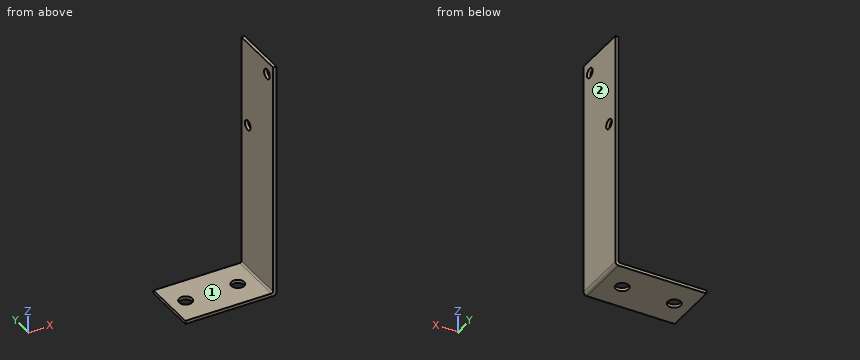
```python
from build123d import *

# Parameters (mm, degrees)
F1_DEPTH = 8.5
F2_R     = 1
F3_R     = 0.5
F4_R     = 2
F5_DEPTH = 3
F6_R     = 1.5
F7_DEPTH = 3


with BuildPart() as f1:
    # F0 (on Front) → F1 (new body, symmetric)
    with BuildSketch(Plane.XZ):
        Polygon((0, 0), (0, 73), (-1, 73), (-1, 1), (-28, 1), (-28, 0), align=None)
    extrude(amount=F1_DEPTH, both=True)

    # F2
    f2_edges = [f1.edges().sort_by_distance(p)[0] for p in [
        (0, 0, 0),
    ]]
    fillet(f2_edges, radius=F2_R)

    # F3
    f3_edges = [f1.edges().sort_by_distance(p)[0] for p in [
        (-1, 0, 1),
    ]]
    fillet(f3_edges, radius=F3_R)

    # F4 (on face) → F5 (cut)
    with BuildSketch(Plane(origin=(0, 0, 0), x_dir=(1, 0, 0), z_dir=(0, 0, -1))):
        with Locations((-23, 0)):
            Circle(F4_R)
        with Locations((-7, 0)):
            Circle(F4_R)
    extrude(amount=-F5_DEPTH, mode=Mode.SUBTRACT)

    # F6 (on face) → F7 (cut)
    with BuildSketch(Plane.YZ):
        with Locations((5.1, 46.8)):
            Circle(F6_R)
        with Locations((-5.15, 69)):
            Circle(F6_R)
    extrude(amount=-F7_DEPTH, mode=Mode.SUBTRACT)


solid = f1.part
```
Here's how the part is built. I have some questions about the finished solid (model axes, mm). Face numbers are marked on the shaded views. A direction names the side the tool comes from. Give positions to 0.01 mm unless a question says otherwise; leave off trailing zeros. Loops run counter-clockwise (first coordinate to the right, second up) from the corner with the lowest first, then second, coordinate; pieces in that order, holes last. Notation, with made-up numbers: M 12.5,85.25 L 43.5,85.25 A29 cw 43.5,111.25 Z; hole C 65.25,9 d4. An arc over 180 degrees is marked long. Put each result on its own line as item: value. Start each with the question number.
(1) I need wall thicknesses on line 1 along Y through (x, z) = (-0.3, 69); line 2 along X through (y, z) = (0, 0.65); line 3 along Y through (x, z) = (-23, 0.8). Which ranges of each line are inside material? Lowest first, please. Write a range as [from, to].
(2) I want a section at C-C on x = -7. Please give me the cut outline in (y, z), then the cut area to 3 significant figures.
(3) I want a section at A-A on z = 46.8. Please give me the cut outline in (x, y).
(4) Will these pins go through, and if not, where does the flat tip stop? pin 1 Ø8.5 at (y, z) = (-3, 51) entering from -X; pin 2 Ø2.5 at (y, z) = (5.1, 46.8) entering from +X; pin 3 Ø5 at (x, y) = (-12.5, 3) entering from +Z; pin 4 Ø5 at (x, y) = (-25, 0.5) entering from -Z.
(5) I want a section at B-B on y = -5.15. Please give me the cut outline in (x, z).
(6) I want a section at D-D on z = 32. Please give me the cut outline in (x, y), then the cut area to 3 significant figures.
(7) For the marked faces 1 and 2, which set-ups out of +Z, -Z, +X, -X, +Y, -Y let a thin tool reach every point of the face, with its end or its side?
Answer block:
1. line 1: [-8.5, -6.65], [-3.65, 8.5]
1. line 2: [-28, -25], [-21, -9], [-5, -0.06]
1. line 3: [-8.5, -2], [2, 8.5]
2. outline: M -8.5,0 L -2,0 L -2,1 L -8.5,1 Z; M 2,0 L 8.5,0 L 8.5,1 L 2,1 Z
2. area: 13.0 mm^2
3. outline: M -1,-8.5 L 0,-8.5 L 0,3.6 L -1,3.6 Z; M -1,6.6 L 0,6.6 L 0,8.5 L -1,8.5 Z
4. pin 1: x = -1
4. pin 2: through
4. pin 3: z = 1
4. pin 4: z = 0
5. outline: M -28,0 L -1,0 A1 ccw 0,1 L 0,67.5 L -1,67.5 L -1,1.5 A0.5 cw -1.5,1 L -28,1 Z; M -1,70.5 L 0,70.5 L 0,73 L -1,73 Z
6. outline: M -1,-8.5 L 0,-8.5 L 0,8.5 L -1,8.5 Z
6. area: 17.0 mm^2
7. face 1: +Z, -X, +Y, -Y
7. face 2: +Z, -Z, +X, +Y, -Y
